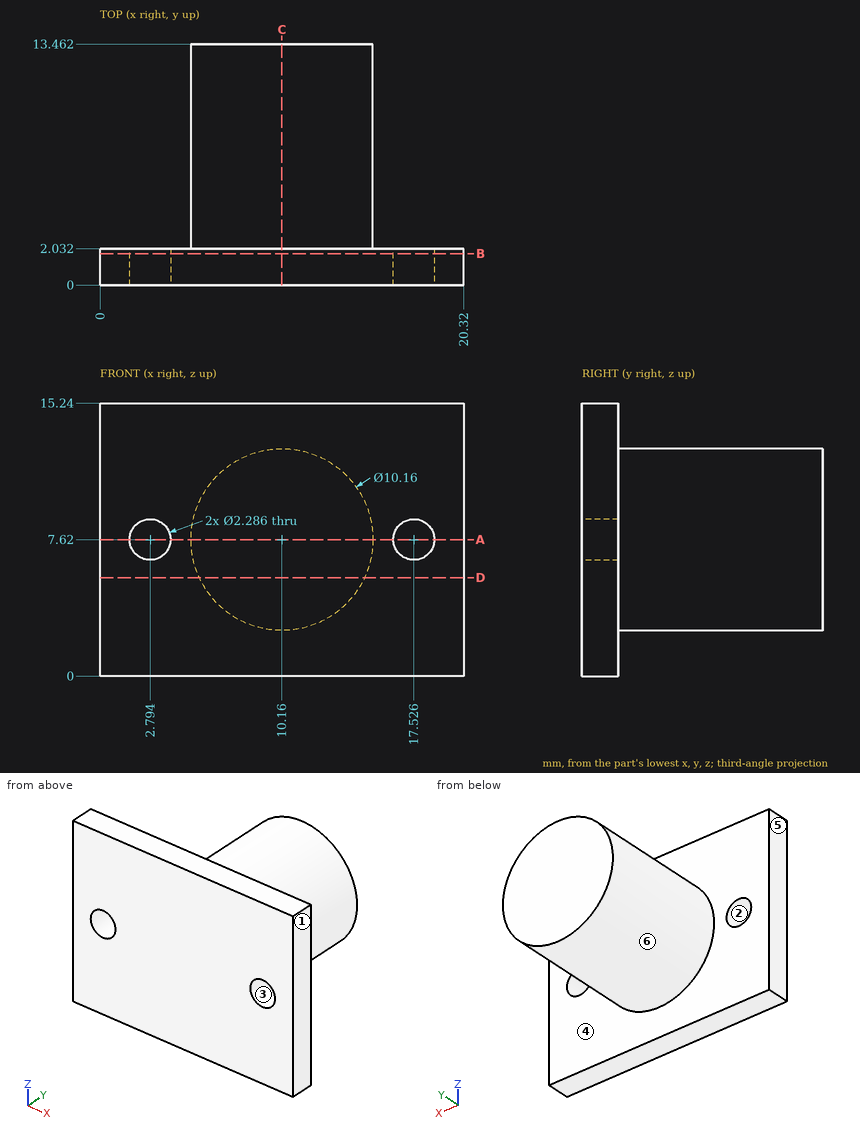
Geometry: see drawing. Coordinates: mm, zero at the bounding-box minimum. A direction names the side the tool comes from. Coordinates: 2 decimals unless noted, no trailing zeros. Loops run counter-clockwise (first coordinate to the right, second up) from the corner with the lowest first, then second, coordinate; pieces in that order, holes last. Notation, with made-up numbers: (-13, 41) - (2, 41) arc R19 ccw to (2, 47) - close; hole circle Ø6 at (-23, -10.75). An arc over 180 degrees is marked (long way). Answer as CSV lines item,"result".
1. Section D-D (z = 5.5). Return loops of the section in (x, y), then the cut area to 3 significant figures.
Established:
outline,"(0, 0) - (20.32, 0) - (20.32, 2.03) - (14.78, 2.03) - (14.78, 13.46) - (5.54, 13.46) - (5.54, 2.03) - (0, 2.03) - close"
area,"147 mm2"
2. Section A-A (z = 7.62). Return loops of the section in (x, y).
Established:
outline,"(0, 0) - (1.65, 0) - (1.65, 2.03) - (0, 2.03) - close; (3.94, 0) - (16.38, 0) - (16.38, 2.03) - (15.24, 2.03) - (15.24, 13.46) - (5.08, 13.46) - (5.08, 2.03) - (3.94, 2.03) - close; (18.67, 0) - (20.32, 0) - (20.32, 2.03) - (18.67, 2.03) - close"
3. Reachability of the marked faces 5 and 6 from +Z, -Z, +X, -X, +Y, -Y: full face, straight path, thin tool, end or side. Return the list, or none.
Established:
face 5,"+Z, -Z, -X, +Y, -Y"
face 6,"+Y"
4. Mould query, pull axis X, two halves, no side actions, for the marked faces 1, 2, 3 and 4. Classes: released by +X, released by -X, zero draft, split by the parting line, or undercut.
Established:
face 1,"released by +X"
face 2,"undercut"
face 3,"undercut"
face 4,"zero draft"
5. Contact query for flat-ended pins moving along their axis: pin 1 (3 mm diameter, centred on x = 14.5, z = 10, fed in from -Y); pin 2 (4 mm diameter, centred on x = 11.5, y = 9.5, fed in from -Z); pin 3 (4 mm diameter, centred on x = 10.5, y = 11, fed in from +Z); pin 4 (6 mm diameter, centred on x = 2.5, z = 4, fed in from +Y). Output: stop coordinate, or through.
Established:
pin 1,"stops at y = 0"
pin 2,"stops at z = 2.54"
pin 3,"stops at z = 12.7"
pin 4,"stops at y = 2.03"
6. Ray query, line 1 (Y direction, x = 2.5, z = 13.5); line 2 (Z direction, x = 14.25, y = 7); line 3 (Z direction, x = 10.25, y = 3.5). Return the intervals inside material, ascending.
Established:
line 1,"y = 0 to 2.03"
line 2,"z = 4.61 to 10.63"
line 3,"z = 2.54 to 12.7"
7. Section B-B (y = 1.75). Return loops of the section in (x, z), then the cut area to 3 significant figures.
Established:
outline,"(0, 0) - (20.32, 0) - (20.32, 15.24) - (0, 15.24) - close; hole circle Ø2.29 at (2.79, 7.62); hole circle Ø2.29 at (17.53, 7.62)"
area,"301 mm2"
8. Section C-C (x = 10.16). Return loops of the section in (y, z).
Established:
outline,"(0, 0) - (2.03, 0) - (2.03, 2.54) - (13.46, 2.54) - (13.46, 12.7) - (2.03, 12.7) - (2.03, 15.24) - (0, 15.24) - close"
